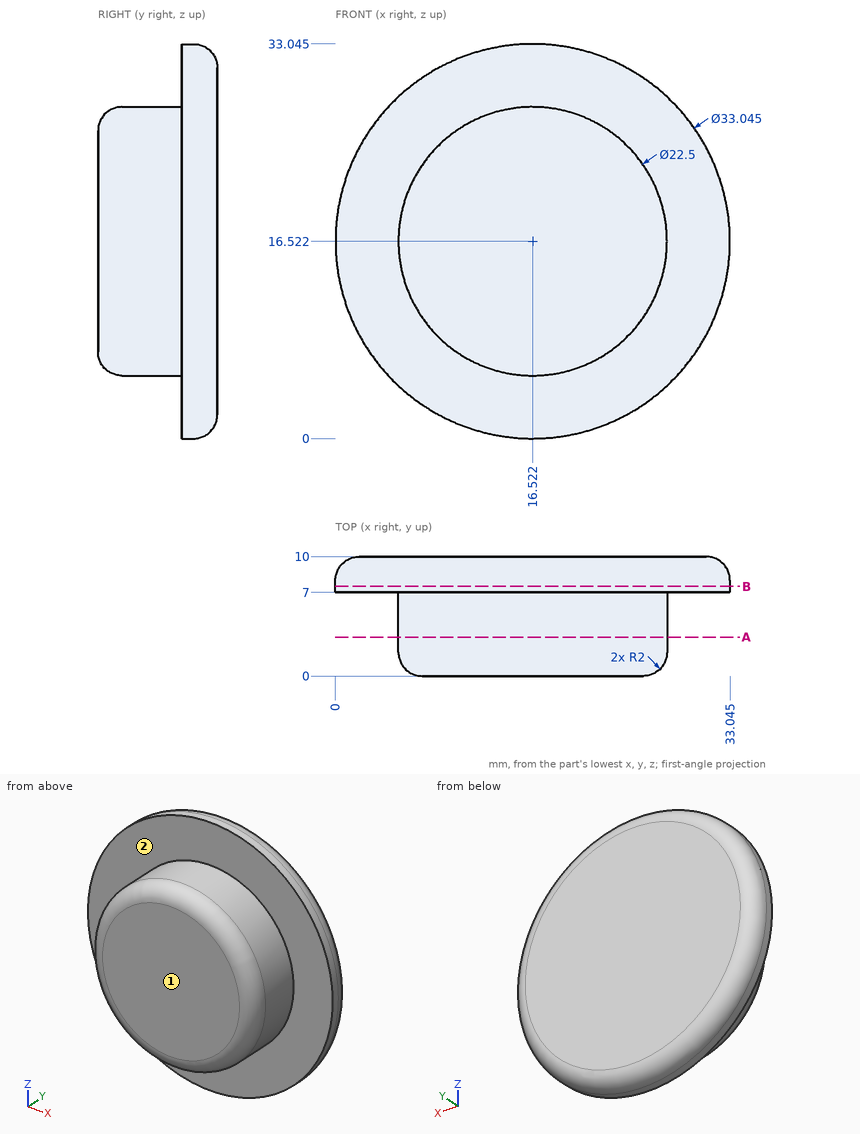
Source: three-view drawing plus pictorial views. Frame: mm from the lowest corner of the part. A direction names the side the tool comes from. Coordinates: 2 decimals unless noted, no trailing zeros. Order: outer loops, then holes, each group sorted by start corner. A loop starts at its lowest first (then second) coordinate and runs counter-clockwise, first axis right, second up. Notation, with made-up numbers: M 59,38.5 L 106,38.5 A7 cw 106,45.5 Z; hole C 67,-26 d10. An arc over 180 degrees is marked long. Answer in a Markdown table with one row per item.
(1) Access query for the marked faces 1 and 2. Directions: +Z, -Z, +X, -X, +Y, -Y. A direction counts if a zero-diameter tool reaches every point of the face in a straight line with its end or side. Return the directions, or none.
Numbers:
| item | result |
|---|---|
| face 1 | +Z, -Z, +X, -X, -Y |
| face 2 | -Y |
(2) Section query A-A, the plane y = 3.25. Output: boundary loops of the cut face in (x, z).
Numbers:
| item | result |
|---|---|
| outline | C 16.52,16.52 d22.5 |
(3) Material intervals for line 1 (Y direction, x = 11.5, z = 30); line 2 (X direction, y = 6, z = 16.5); line 3 (Z direction, x = 19.5, y = 6.75), sorted ascending. Write a range as [from, to].
Numbers:
| item | result |
|---|---|
| line 1 | y = [7, 10] |
| line 2 | x = [5.27, 27.77] |
| line 3 | z = [5.67, 27.37] |
(4) Section query B-B, the plane y = 7.5. Output: boundary loops of the cut face in (x, z) (1 decimal).
Numbers:
| item | result |
|---|---|
| outline | C 16.5,16.5 d33 |
(5) Contact query for flat-ended pins moving along their axis: pin 1 Ø2 at (x, z) = (26.5, 8.5) entering from -Y; pin 2 Ø5 at (x, y) = (15, 4) entering from +Z; pin 3 Ø1.5 at (x, y) = (24, 8) entering from +Z. Output: stop coordinate, or through.
Numbers:
| item | result |
|---|---|
| pin 1 | stops at y = 7 |
| pin 2 | stops at z = 27.77 |
| pin 3 | stops at z = 31.61 |
